Work out the finished part from the listing and answer in its coordinate system (mm). Face numbers are marked on the shaded views. Give positions to 0.01 mm unless a question says otherwise; leave off trailing zeros. Loops run counter-clockwise (first coordinate to the right, second up) from the corner with the lowest first, then second, coordinate; pieces in that order, holes last. Notation, with made-up numbers: M -19,56.25 L 25,56.25 A21 cw 25,79.25 Z; hole C 77,-22 d1. An arc over 180 degrees is marked long. Write item = value, one per line. Start each with the question number.
1. Section A-A on z = 12.75 is taken. Determine the outline of the cut face in (x, y) (3 decimals), plus the area to 3 significant figures.
2. Flat-ended cylindrical pins translate along their axes: pin 1 Ø8 at (y, z) = (53, 3) entering from +X; pin 2 Ø1.5 at (x, y) = (-5.5, 31) entering from +Z; pin 3 Ø3 at (y, z) = (22.5, 4.5) entering from -X. Find the tip coordinate at first contact, or state that the pin passes through.
3. Section C-C on y = -3.5 is taken. Determine the outline of the cut face in (x, z), plus the area to 3 significant figures.
4. The mould has two halves that part along X. Classify the marked faces 1, 2 and 3: released by +X, released by -X, zero draft, split by the parting line, or undercut.
5. Section D-D on y = 72 is taken. Determine the outline of the cut face in (x, z).
6. Consider L1, parallel to Z at x = -4.75, y = 78; L2, parallel to Z at x = -6, y = 43; L3, parallel to Y at x = -4.75, z = 8.5. Determine where each line is inside the solid, lowest interval first. Write a range as [from, to].
7. Section B-B on x = -4 is taken. Determine the outline of the cut face in (y, z), plus the area to 3 significant figures.
```python
from build123d import *

# Parameters (mm, degrees)
F1_DEPTH      = 6.35
F2_DEPTH      = 19.05
F3_DEPTH      = 6.35
F5_DEPTH      = 25.4
F5_DEPTH_BACK = 25.4


with BuildPart() as f1:
    # F0 (on Top) → F1 (new body)
    with BuildSketch(Plane.XY):
        with BuildLine():
            Line((-9.4939634524, 93.546902302), (-5.715, 0))
            Line((-5.715, 0), (0, -13.6347989514))
            Line((0, -13.6347989514), (5.715, 0))
            Line((5.715, 0), (9.4939634524, 93.546902302))
            ThreePointArc((9.4939634524, 93.546902302), (0, 84.7902010486), (-9.4939634524, 93.546902302))
        make_face()
    extrude(amount=F1_DEPTH)

    # F0 (on Top) → F2 (join)
    with BuildSketch(Plane.XY):
        with BuildLine():
            Line((-9.525, 94.3152010486), (-9.4939634524, 93.546902302))
            ThreePointArc((-9.4939634524, 93.546902302), (0, 84.7902010486), (9.4939634524, 93.546902302))
            Line((9.4939634524, 93.546902302), (9.525, 94.3152010486))
            Line((9.525, 94.3152010486), (6.35, 94.3152010486))
            ThreePointArc((6.35, 94.3152010486), (0, 87.9652010486), (-6.35, 94.3152010486))
            Line((-6.35, 94.3152010486), (-9.525, 94.3152010486))
        make_face()
    extrude(amount=F2_DEPTH)

    # F3 (add): faces of the model
    f3_faces = [f1.faces().sort_by_distance(p)[0] for p in [
        (-7.9375, 94.3152010486, 9.525),
        (7.9375, 94.3152010486, 9.525),
    ]]
    extrude(f3_faces, amount=F3_DEPTH)

    # F4 (on Right) → F5 (cut, two sides)
    with BuildSketch(Plane.YZ) as f5_sk:
        Polygon((-30.6564283764, 9.0817261184), (-14.1004319647, 2.4969553254), (49.8651257087, 6.4478169652), (49.8651257087, 26.7665392731), align=None)
    extrude(amount=-F5_DEPTH, mode=Mode.SUBTRACT)
    extrude(f5_sk.sketch, amount=F5_DEPTH_BACK, mode=Mode.SUBTRACT)


solid = f1.part
```
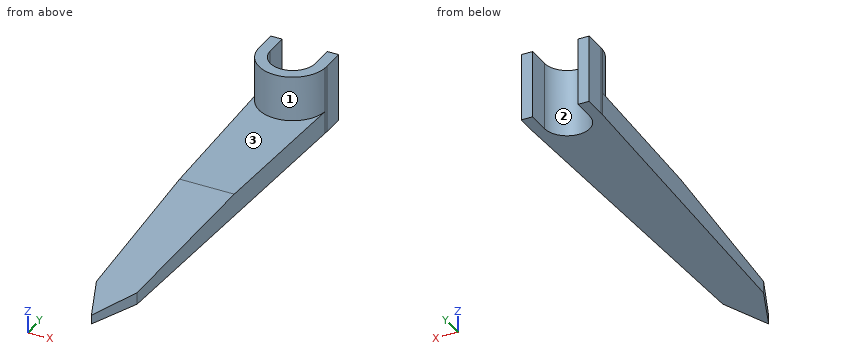
Verdict:
q1.outline = M -9.525,94.315 L -9.494,93.547 A9.525 ccw 9.494,93.547 L 9.525,94.315 L 9.525,100.665 L 6.35,100.665 L 6.35,94.315 A6.35 cw -6.35,94.315 L -6.35,100.665 L -9.525,100.665 Z
q1.area = 119 mm2
q2.pin_1 = 8.02
q2.pin_2 = 5.33
q2.pin_3 = -6.68
q3.outline = M -4.25,0 L 4.25,0 L 4.25,3.15 L -4.25,3.15 Z
q3.area = 26.8 mm2
q4.face_1 = split by the parting line
q4.face_2 = undercut
q4.face_3 = zero draft
q5.outline = M -8.62,0 L 8.62,0 L 8.62,6.35 L -8.62,6.35 Z
q6.L1 = [0, 6.35]
q6.L2 = [0, 6.02]
q6.L3 = [86.06, 90.1]
q7.outline = M -4.09,0 L 89.38,0 L 89.38,19.05 L 85.67,19.05 L 85.67,6.35 L 48.28,6.35 L -4.09,3.12 Z
q7.area = 556 mm2
